Job drawing, mm, ordinate dimensions from the low corner. One solid piece. A direction names the side the tool comes from. Coordinates: 2 decimals unless noted, no trailing zeros. Write each loop counter-clockwise with the first axis right and the second up, starting at its lowest first coordinate (ties: lowest second). Pieces come first, ordered by that corner, then holes. Notation, with made-up numbers: (68.5, 43) - (97.5, 43) arc R19 ccw to (97.5, 74) - close; hole circle Ø4 at (58.25, 15). An arc over 180 degrees is marked (long way). Put each result on its own line as item: value. Start each with the question number.
1. Saw through at B-B, the plane x = 23.5. Write the cut outline in (y, z), plus the area to 3 significant figures.
2. Saw through at A-A, the plane z = 29. Write the cut outline in (x, y).
3. Saw through at C-C, the plane y = 41. Write the cut outline in (x, z).
4. Pull direction Z, two halves, no side cores. Call the marked faces 3, 4, 5 and 6: released by +Z, released by -Z, zero draft, split by the parting line, or undercut.
5. Drop flat-ended pins along their axis: P1, Ø4, axis at x = 96.5, y = 34.5, coming from the +Z side; P2, Ø1.5, axis at x = 130, y = 18.5, coming from the +Z side; P3, Ø4, axis at y = 20.5, z = 41.5, coming from the +X side. Give the stop position or say it passes through.
6. Drill centre lines: L1, parallel to X at y = 34, z = 38; L2, parallel to Z at x = 14.5, y = 5; L3, parallel to Z at x = 120, y = 8. Where is each one in solid material? Low to high. Write a range as from..to.
7. Saw through at D-D, the plane x = 123.5. Write the cut outline in (y, z), plus the area to 3 significant figures.
8. Which spindle directions (+Z, -Z, +X, -X, +Y, -Y) get a long thin tool onto all of the face, cutting with end or side? Do the marked faces 1 and 2. Say none if no direction does.
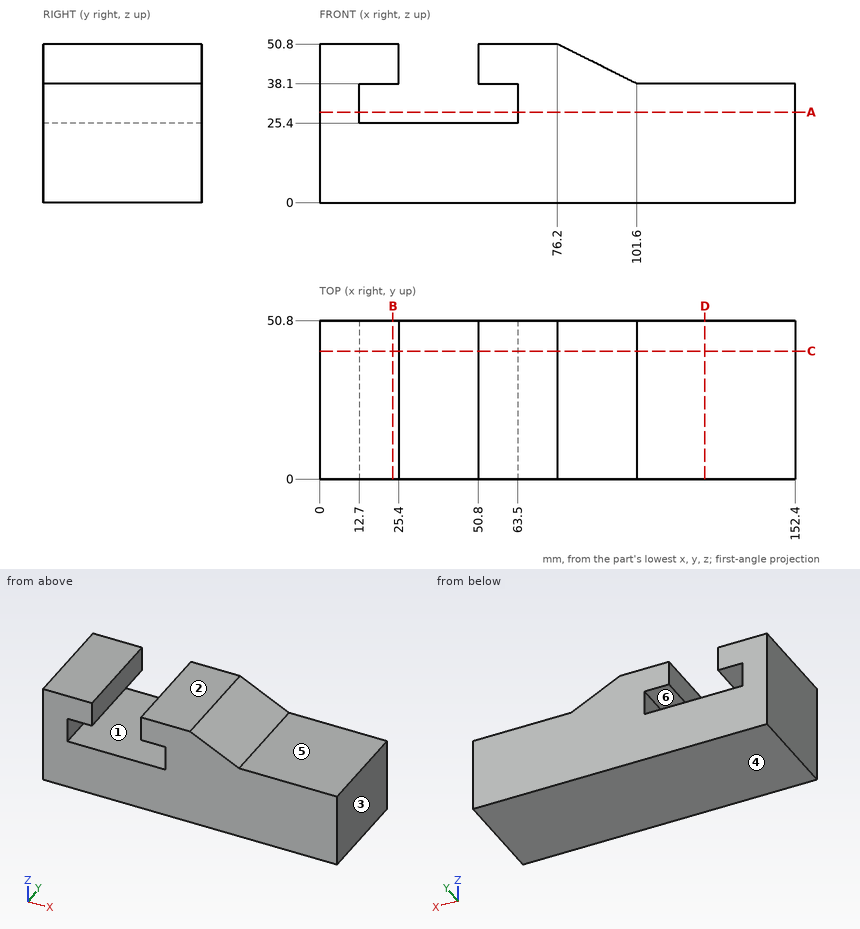
Final values:
1. outline: (0, 0) - (50.8, 0) - (50.8, 25.4) - (0, 25.4) - close; (0, 38.1) - (50.8, 38.1) - (50.8, 50.8) - (0, 50.8) - close
1. area: 1,940 mm²
2. outline: (0, 0) - (12.7, 0) - (12.7, 50.8) - (0, 50.8) - close; (63.5, 0) - (152.4, 0) - (152.4, 50.8) - (63.5, 50.8) - close
3. outline: (0, 0) - (152.4, 0) - (152.4, 38.1) - (101.6, 38.1) - (76.2, 50.8) - (50.8, 50.8) - (50.8, 38.1) - (63.5, 38.1) - (63.5, 25.4) - (12.7, 25.4) - (12.7, 38.1) - (25.4, 38.1) - (25.4, 50.8) - (0, 50.8) - close
4. face 3: zero draft
4. face 4: released by -Z
4. face 5: released by +Z
4. face 6: undercut
5. P1: stops at z = 41.65
5. P2: stops at z = 38.1
5. P3: stops at x = 98.8
6. L1: x = 0..12.7, 63.5..152.4
6. L2: z = 0..25.4, 38.1..50.8
6. L3: z = 0..38.1
7. outline: (0, 0) - (50.8, 0) - (50.8, 38.1) - (0, 38.1) - close
7. area: 1,940 mm²
8. face 1: +Y, -Y
8. face 2: +Z, +X, -X, +Y, -Y
